The listing builds one solid part. Answer for the finished solid, in the listing's coordinates (mm). Give positions to 0.01 mm unless a question says otherwise; leave off trailing zeros. Write each loop counter-clockwise with the first axis right and the second up, starting at its lowest first coordinate (ties: lowest second). Pieces come first, ordered by that corner, then holes. Notation, with made-up numbers: M -37,31.5 L -3,31.5 A19 cw -3,35.5 Z; hole C -7,41 d8. An arc over 180 degrees is marked long. Return JSON: item names as keys, results as strings.
Autodesk Inventor part; units mm, degrees
ref_plane "YZ Plane" through (0, 0, 0) normal (1, 0, 0) x (0, 1, 0)
ref_plane "XZ Plane" through (0, 0, 0) normal (0, 1, 0) x (-1, 0, 0)
ref_plane "XY Plane" through (0, 0, 0) normal (0, 0, 1) x (1, 0, 0)
sketch "Boceto1" plane through (0, 0, 0) normal (0, 1, 0) x (-1, 0, 0)
  circle A0 centre (4.7317, 15.3673) radius 6
  point P0 (0, 0)
  dimension "d0" = 12
extrude "Extrusión1" add sketch "Boceto1" along normal blind 434
thread "Rosca1"
sketch "Sketch2" plane through (-4.7317, 0, 15.3673) normal (0, -1, 0) x (1, 0, 0)
  circle A0 centre (0, 0) radius 4
  circle A1 centre (0, 0) radius 6
  dimension "d5" = 8
extrude "Extrusion2" cut sketch "Sketch2" against normal blind 12
sketch "Sketch3" plane through (-4.7317, 434, 15.3673) normal (0, 1, 0) x (1, 0, 0)
  circle A0 centre (0, 0) radius 5
  circle A1 centre (0, 0) radius 6
  dimension "d8" = 10
extrude "Extrusion3" cut sketch "Sketch3" against normal blind 10
properties part number "Tornillo de mesa" material "Steel"
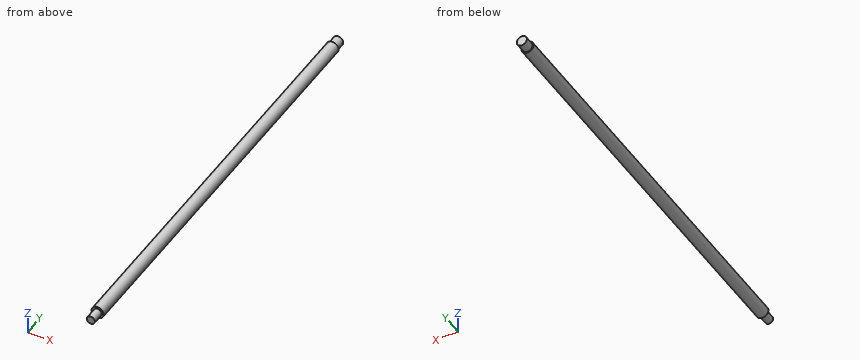
Item 1: A cutting plane is placed at B-B, the plane y = 257. Write down the section's boundary in (x, z), plus the area to 3 significant figures.
Geometry results:
{"outline": "C -4.73,15.37 d12", "area": "113 mm2"}
Item 2: A cutting plane is placed at A-A, the plane x = -4. Write down the section's boundary in (y, z), plus the area to 3 significant figures.
Geometry results:
{"outline": "M 0,11.43 L 12,11.43 L 12,9.41 L 424,9.41 L 424,10.42 L 434,10.42 L 434,20.31 L 424,20.31 L 424,21.32 L 12,21.32 L 12,19.3 L 0,19.3 Z", "area": "5,100 mm2"}
Item 3: Find the intervals of material crossed by line 1 (Y direction, x = -2.25, z = 20.75); line 2 (Y direction, x = -5.5, z = 10.75); line 3 (Z direction, x = -5.5, y = 274.5), in increasing order.
Geometry results:
{"line 1": "y = 12 to 424", "line 2": "y = 12 to 434", "line 3": "z = 9.42 to 21.32"}
Item 4: Given pin 1 Ø5 at (x, y) = (-3.5, 364) entering from +Z; pin 2 Ø1 at (y, z) = (241.5, 11.5) entering from -X; pin 3 Ø2 at (y, z) = (213.5, 14) entering from +X; pin 4 Ø5 at (x, y) = (-8.5, 256.5) entering from -Z, each flat-ended and moving along its own axis, determine where each tip first touches the part or whether it passes through.
Geometry results:
{"pin 1": "stops at z = 21.37", "pin 2": "stops at x = -9.7", "pin 3": "stops at x = 1.26", "pin 4": "stops at z = 9.5"}
